from build123d import *

# Parameters (mm, degrees)
DODANIE_WYCI_GNI_CIE1_DEPTH = 1
SZKIC12_W                   = 9.1
SZKIC12_H                   = 7
DODANIE_WYCI_GNI_CIE2_DEPTH = 1
SZKIC15_W                   = 1.5
SZKIC15_H                   = 7
DODANIE_WYCI_GNI_CIE3_DEPTH = 3
WYTNIJ_WYCI_GNI_CIE1_DEPTH  = 1


with BuildPart() as part:
    # Szkic1 → Dodanie-wyciągnięcie1 (new body)
    with BuildSketch(Plane.XY):
        with BuildLine():
            Line((-7.206635208, 4.522640333), (-7.206635208, -2.477359667))
            Line((-7.206635208, -2.477359667), (15.793364792, -2.477359667))
            Line((15.793364792, -2.477359667), (15.793364792, -0.577359667))
            Line((15.793364792, -0.577359667), (13.620412834, -0.577359667))
            Line((13.620412834, -0.577359667), (12.700412834, -0.577359667))
            ThreePointArc((12.700412834, -0.577359667), (11.100412834, 1.022640333), (12.700412834, 2.622640333))
            Line((12.700412834, 2.622640333), (13.620412834, 2.622640333))
            Line((13.620412834, 2.622640333), (15.793364792, 2.622640333))
            Line((15.793364792, 2.622640333), (15.793364792, 4.522640333))
            Line((15.793364792, 4.522640333), (-7.206635208, 4.522640333))
        make_face()
    extrude(amount=DODANIE_WYCI_GNI_CIE1_DEPTH)

    # Szkic12 → Dodanie-wyciągnięcie2 (add)
    with BuildSketch(Plane.ZY.offset(7.206635208)):
        with Locations((4.55, 1.022640333)):
            Rectangle(SZKIC12_W, SZKIC12_H)
    extrude(amount=-DODANIE_WYCI_GNI_CIE2_DEPTH)

    # Szkic15 → Dodanie-wyciągnięcie3 (add)
    with BuildSketch(Plane.ZY.offset(7.206635208)):
        with Locations((9.85, 1.022640333)):
            Rectangle(SZKIC15_W, SZKIC15_H)
    extrude(amount=-DODANIE_WYCI_GNI_CIE3_DEPTH)

    # Szkic16 → Wytnij-wyciągnięcie1 (cut)
    with BuildSketch(Plane(origin=(-6.206635208, 0, 0), x_dir=(0, 0, -1), z_dir=(1, 0, 0))):
        with BuildLine():
            Line((-7.5, -0.577359667), (-5, -0.577359667))
            ThreePointArc((-5, -0.577359667), (-3.4, 1.022640333), (-5, 2.622640333))
            Line((-5, 2.622640333), (-7.5, 2.622640333))
            ThreePointArc((-7.5, 2.622640333), (-9.1, 1.022640333), (-7.5, -0.577359667))
        make_face()
    extrude(amount=-WYTNIJ_WYCI_GNI_CIE1_DEPTH, mode=Mode.SUBTRACT)


solid = part.part
Check sheet for the modelled part. Datum: model origin and axes. Units: mm. A direction names the side the tool comes from. Round coordinates to 2 decimals unless told otherwise and drop trailing zeros. Loops run counter-clockwise (first coordinate to the right, second up) from the corner with the lowest first, then second, coordinate; pieces in that order, holes last. Notation, with made-up numbers: M -27.75,38 L 25.25,38 A6 cw 25.25,47 Z; hole C 46,0.25 d11. An arc over 180 degrees is marked long. One line per question, with ' | ' between items. Start each with the question number.
Item 1: Section check B-B (z = 5.75). Record the boundary of the cut face in (x, y), and give its area (3 significant figures).
Item 2: Section check C-C (y = -1.5). Record the boundary of the cut face in (x, z), and give its area (3 significant figures).
Item 3: Set-up check for faces 1 (the face through (14.2, 2.623, 0.5)), 2 (the face through (-5, 1, 9.1)), 3 (the face through (-4.207, 1, 10)): record each of +Z, -Z, +X, -X, +Y, -Y from which the full face is reachable in a straight line by a thin tool's end or side.
Item 4: Scan lines: probe 1 along Z at (x, y) = (-6, 4); probe 2 along X at (y, z) = (4, 8.25); probe 3 along Z at (x, y) = (3.5, 2). Record each from-to range of solid material in increasing order.
Item 5: Gauge pin test, flat ends, axial feed: pin 1 Ø2 at (x, y) = (9, 0.5) entering from +Z; pin 2 Ø1.2 at (y, z) = (1.5, 9.5) entering from +X; pin 3 Ø2 at (y, z) = (-0.5, 4) entering from +X. Record the tip position at first contact, or that the pin passes through.
Item 6: Section check A-A (x = 13). Record the boundary of the cut face in (y, z).
Item 7: Section check D-D (y = -0.25). Record the boundary of the cut face in (x, z), and give its area (3 significant figures).
Worked out:
1) outline: M -7.21,-2.48 L -6.21,-2.48 L -6.21,-0.58 L -7.21,-0.58 Z; M -7.21,2.62 L -6.21,2.62 L -6.21,4.52 L -7.21,4.52 Z | area: 3.80 mm^2
2) outline: M -7.21,0 L 15.79,0 L 15.79,1 L -6.21,1 L -6.21,9.1 L -4.21,9.1 L -4.21,10.6 L -7.21,10.6 Z | area: 35.6 mm^2
3) face 1: +Z, -Z, +X | face 2: +X, +Y, -Y | face 3: +Z, +X, +Y, -Y
4) probe 1: 0 to 1, 9.1 to 10.6 | probe 2: -7.21 to -6.21 | probe 3: 0 to 1
5) pin 1: z = 1 | pin 2: x = -4.21 | pin 3: x = -6.21
6) outline: M -2.48,0 L -0.58,0 L -0.58,1 L -2.48,1 Z; M 2.62,0 L 4.52,0 L 4.52,1 L 2.62,1 Z
7) outline: M -7.21,0 L 11.73,0 L 11.73,1 L -6.21,1 L -6.21,4.03 L -7.21,4.03 Z; M -7.21,8.47 L -6.21,8.47 L -6.21,9.1 L -4.21,9.1 L -4.21,10.6 L -7.21,10.6 Z | area: 27.1 mm^2
